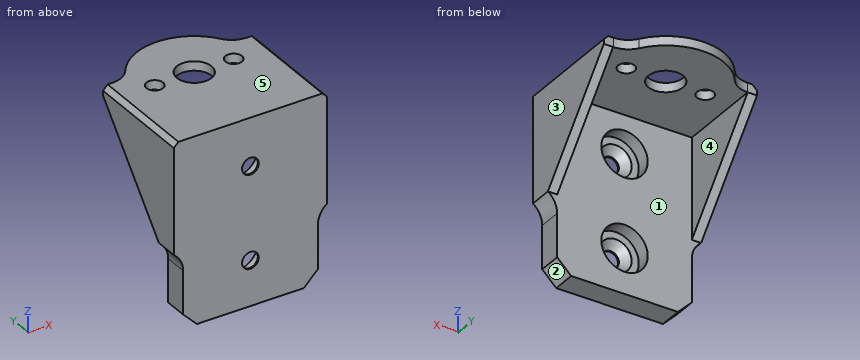
from build123d import *

# Parameters (mm, degrees)
SKETCH1_W                                    = 23
SKETCH1_H                                    = 40
SKETCH1_R                                    = 1.75
BOSS_EXTRUDE1_DEPTH                          = 5
SKETCH2_W                                    = 23
SKETCH2_H                                    = 2
BOSS_EXTRUDE2_DEPTH                          = 50
SKETCH3_R                                    = 1.8
SKETCH3_R_2                                  = 3.75
CUT_EXTRUDE1_DEPTH                           = 69.972820734
BOSS_EXTRUDE3_DEPTH                          = 3
BOSS_EXTRUDE4_START                          = -23
BOSS_EXTRUDE4_DEPTH                          = 3
BOSS_EXTRUDE5_DEPTH                          = 2
BOSS_EXTRUDE6_START                          = -29
BOSS_EXTRUDE6_DEPTH                          = 2
SKETCH6_R                                    = 5
CUT_EXTRUDE2_DEPTH                           = 3
CSK_FOR_M3_HEX_SOCKET_COUNTERSUNK_HE_2_COUNT = 2
CSK_FOR_M3_HEX_SOCKET_COUNTERSUNK_HE_2_PITCH = 20
CHAMFER1_SIZE                                = 3
CHAMFER2_SIZE                                = 1
FILLET1_R                                    = 5


with BuildPart() as part:
    # Sketch1 → Boss-Extrude1 (new body)
    with BuildSketch(Plane(origin=(0, 0, 0), x_dir=(1, 0, 0), z_dir=(0, 1, 0))):
        with Locations((0, -10.3)):
            Rectangle(SKETCH1_W, SKETCH1_H)
        with Locations(Location((0, 0, 0), (0, 0, 270))):
            Circle(SKETCH1_R, mode=Mode.SUBTRACT)
        with Locations(Location((0, -20, 0), (0, 0, 270))):
            Circle(SKETCH1_R, mode=Mode.SUBTRACT)
    extrude(amount=BOSS_EXTRUDE1_DEPTH)

    # Sketch2 → Boss-Extrude2 (add)
    with BuildSketch(Plane(origin=(0, 5, 0), x_dir=(1, 0, 0), z_dir=(0, 1, 0))):
        with Locations((0, -29.3)):
            Rectangle(SKETCH2_W, SKETCH2_H)
    extrude(amount=BOSS_EXTRUDE2_DEPTH)

    # Sketch3 → Cut-Extrude1 (cut, through all)
    with BuildSketch(Plane.XY.offset(30.3)):
        with Locations((-8.5, 18.8)):
            Circle(SKETCH3_R)
        with Locations((8.5, 18.8)):
            Circle(SKETCH3_R)
        with Locations((0, 18.8)):
            Circle(SKETCH3_R_2)
        with BuildLine():
            Line((-11.5, 23.698979486), (-11.5, 55))
            Line((-11.5, 55), (11.5, 55))
            Line((11.5, 55), (11.5, 23.698979486))
            ThreePointArc((11.5, 23.698979486), (0, 31.3), (-11.5, 23.698979486))
        make_face()
    extrude(amount=-CUT_EXTRUDE1_DEPTH, mode=Mode.SUBTRACT)

    # Sketch4 → Boss-Extrude3 (add)
    with BuildSketch(Plane.ZY.offset(11.5)):
        Polygon((30.3, 0), (30.3, 23.698979486), (28.3, 23.698979486), (28.3, 5), (-9.7, 5), (-9.7, 0), align=None)
    extrude(amount=BOSS_EXTRUDE3_DEPTH)

    # Sketch4<2> → Boss-Extrude4 (add)
    with BuildSketch(Plane.ZY.offset(11.5).offset(BOSS_EXTRUDE4_START)):
        Polygon((30.3, 0), (30.3, 23.698979486), (28.3, 23.698979486), (28.3, 5), (-9.7, 5), (-9.7, 0), align=None)
    extrude(amount=-BOSS_EXTRUDE4_DEPTH)

    # Sketch5 → Boss-Extrude5 (add)
    with BuildSketch(Plane(origin=(14.5, 0, 0), x_dir=(0, 0, -1), z_dir=(1, 0, 0))):
        Polygon((-30.3, 23.698979486), (-30.3, 0), (-6.601020514, 0), (-6.601020514, 5), (-28.3, 23.698979486), align=None)
    extrude(amount=BOSS_EXTRUDE5_DEPTH)

    # Sketch5<2> → Boss-Extrude6 (add)
    with BuildSketch(Plane(origin=(14.5, 0, 0), x_dir=(0, 0, -1), z_dir=(1, 0, 0)).offset(BOSS_EXTRUDE6_START)):
        Polygon((-30.3, 23.698979486), (-30.3, 0), (-6.601020514, 0), (-6.601020514, 5), (-28.3, 23.698979486), align=None)
    extrude(amount=-BOSS_EXTRUDE6_DEPTH)

    # Sketch6 → Cut-Extrude2 (cut)
    with BuildSketch(Plane(origin=(0, 5, 0), x_dir=(1, 0, 0), z_dir=(0, 1, 0))):
        with Locations(Location((0, 0, 0), (0, 0, 270))):
            Circle(SKETCH6_R)
        with Locations(Location((0, -20, 0), (0, 0, 270))):
            Circle(SKETCH6_R)
    extrude(amount=-CUT_EXTRUDE2_DEPTH, mode=Mode.SUBTRACT)

    # Sketch8 → CSK for M3 Hex Socket Countersunk Head Screw1 (revolve, cut)
    with BuildSketch(Plane(origin=(0, 2, 0), x_dir=(0, 0, 1), z_dir=(1, 0, 0))):
        Polygon((0, 0), (0, 2), (1.8, 2), (1.8, 1.67), (3.47, 0), align=None)
    csk_for_m3_hex_socket_countersunk_head_s = revolve(axis=Axis((0, 8.35, 0), (0, -1, 0)), mode=Mode.SUBTRACT)

    # CSK for M3 Hex Socket Countersunk He 2: CSK for M3 Hex Socket Countersunk Head Screw1 ×2
    with Locations(*[(0, 0, i * CSK_FOR_M3_HEX_SOCKET_COUNTERSUNK_HE_2_PITCH) for i in range(1, CSK_FOR_M3_HEX_SOCKET_COUNTERSUNK_HE_2_COUNT)]):
        add(csk_for_m3_hex_socket_countersunk_head_s, mode=Mode.SUBTRACT)

    # Chamfer1
    chamfer1_edges = [part.edges().sort_by_distance(p)[0] for p in [
        (-14.5, 2.5, -9.7),
        (14.5, 2.5, -9.7),
    ]]
    chamfer(chamfer1_edges, length=CHAMFER1_SIZE)

    # Chamfer2
    chamfer2_edges = [part.edges().sort_by_distance(p)[0] for p in [
        (16.5, 11.849489743, 30.3),
        (-16.5, 11.849489743, 30.3),
    ]]
    chamfer(chamfer2_edges, length=CHAMFER2_SIZE)

    # Fillet1
    # the kernel refuses this fillet: 5 mm, written as the material it adds along each edge
    with BuildSketch(Plane(origin=(11.5, 23.698979486, 30.3), x_dir=(1, 0, 0), z_dir=(0, 0, -1))) as fillet1_piece_1:
        with BuildLine():
            CenterArc((2.931223273, -5), FILLET1_R, 90, 55.552144514)
            ThreePointArc((-1.191983377, -2.171720147), (-0.54205816, -1.115462354), (0, 0))
            Line((0, 0), (2.931223273, 0))
        make_face()
    extrude(amount=2)
    with BuildSketch(Plane(origin=(-11.5, 23.698979486, 30.3), x_dir=(-1, 0, 0), z_dir=(0, 0, -1))) as fillet1_piece_2:
        with BuildLine():
            CenterArc((2.931223273, 5), FILLET1_R, 214.447855486, 55.552144514)
            ThreePointArc((-1.191983377, 2.171720147), (-0.54205816, 1.115462354), (0, 0))
            Line((0, 0), (2.931223273, 0))
        make_face()
    extrude(amount=2)
    with BuildSketch(Plane(origin=(-14.5, 0, 6.601020514), x_dir=(-1, 0, 0), z_dir=(0, 1, 0))) as fillet1_piece_3:
        with BuildLine():
            CenterArc((5, -4), FILLET1_R, 126.869897646, 53.130102354)
            Line((0, -4), (0, 0))
            Line((0, 0), (2, 0))
        make_face()
    extrude(amount=5)
    with BuildSketch(Plane(origin=(14.5, 0, 6.601020514), x_dir=(1, 0, 0), z_dir=(0, 1, 0))) as fillet1_piece_4:
        with BuildLine():
            CenterArc((5, 4), FILLET1_R, 180, 53.130102354)
            Line((0, 4), (0, 0))
            Line((0, 0), (2, 0))
        make_face()
    extrude(amount=5)


solid = part.part
Read the model definition and answer for the solid it produces. Units are mm, in the model's axes. Face numbers are marked on the shaded views. A direction names the side the tool comes from. Give positions to 0.01 mm unless a question says otherwise; leave off trailing zeros. Write each loop counter-clockwise with the first axis right and the second up, starting at its lowest first coordinate (ties: lowest second). Pieces come first, ordered by that corner, then holes. Notation, with made-up numbers: (-26, 27) -> (17, 27) arc R28 cw to (17, 58) -> close; hole circle Ø11 at (74.25, 4.25). An arc over 180 degrees is marked (long way). Answer as a JSON object with one key per item and string values. Group by question number.
1) Find section A-A (y = 18.8). Write down the section's boundary in (x, z), and give its area (3 significant figures).
2) Find section D-D (z = 13.5). Write down the section's boundary in (x, y).
3) Find section B-B (x = 8.5). Write down the section's boundary in (y, z), and give its area (3 significant figures).
4) Consider L1, parallel to Z at x = 0, y = 0.2; L2, parallel to X at y = 0.15, z = 0; L3, parallel to Z at x = -2.5, y = 2.5. Determine where each line is inside the solid, lowest interval first. Write a range as from..to.
5) A tool of negligible diameter and unlimited length cuts with its end or side. For the marked faces 1 and 2, from which of +Z, -Z, +X, -X, +Y, -Y can it reach the whole face along a straight path? Write none if from no direction.
6) The mould has two halves that part along X. Classify the marked faces 3, 4 and 5: +X half, -X half, draft (parallel to the pull), parting line (faces both ways), or undercut.
7) Find section C-C (z = 20). Write down the section's boundary in (x, y).
8) Each of these flat-tipped pins is pushed along its axis until it touches: P1, Ø2, axis at x = 15, z = 29.5, coming from the +Y side; P2, Ø5.5, axis at y = 3.5, z = -2.5, coming from the +X side; P3, Ø3, axis at x = 8.5, y = 18.8, coming from the -Z side; P4, Ø6, axis at x = 4, y = 22.5, coming from the -Z side. Where does it stop, or does it pass through?
Values follow:
{
 "1": {"outline": "(-16.5, 22.62) -> (-14.5, 22.62) -> (-14.5, 28.3) -> (-10.3, 28.3) -> (-10.3, 30.3) -> (-15.5, 30.3) -> (-16.5, 29.3) -> close; (-6.7, 28.3) -> (-3.75, 28.3) -> (-3.75, 30.3) -> (-6.7, 30.3) -> close; (3.75, 28.3) -> (6.7, 28.3) -> (6.7, 30.3) -> (3.75, 30.3) -> close; (10.3, 28.3) -> (14.5, 28.3) -> (14.5, 22.62) -> (16.5, 22.62) -> (16.5, 29.3) -> (15.5, 30.3) -> (10.3, 30.3) -> close", "area": "58.3 mm2"},
 "2": {"outline": "(-16.5, 0) -> (16.5, 0) -> (16.5, 10.95) -> (14.5, 10.95) -> (14.5, 5) -> (-14.5, 5) -> (-14.5, 10.95) -> (-16.5, 10.95) -> close"},
 "3": {"outline": "(0, -9.7) -> (5, -9.7) -> (5, 28.3) -> (17, 28.3) -> (17, 30.3) -> (0, 30.3) -> close; (20.6, 28.3) -> (27.97, 28.3) -> (27.97, 30.3) -> (20.6, 30.3) -> close", "area": "239 mm2"},
 "4": {"L1": "z = -9.7..-1.8, 1.8..18.2, 21.8..30.3", "L2": "x = -14.5..-1.8, 1.8..14.5", "L3": "z = -9.7..-4.33, 4.33..15.67, 24.33..30.3"},
 "5": {"face 1": "-Z, +Y", "face 2": "-Z, +X, +Y, -Y"},
 "6": {"face 3": "+X half", "face 4": "undercut", "face 5": "draft"},
 "7": {"outline": "(-16.5, 0) -> (-1.8, 0) -> (-1.8, 0.33) -> (-3.47, 2) -> (-5, 2) -> (-5, 5) -> (-14.5, 5) -> (-14.5, 16.55) -> (-16.5, 16.55) -> close; (1.8, 0) -> (16.5, 0) -> (16.5, 16.55) -> (14.5, 16.55) -> (14.5, 5) -> (5, 5) -> (5, 2) -> (3.47, 2) -> (1.8, 0.33) -> close"},
 "8": {"P1": "stops at y = 23.72", "P2": "stops at x = 14.5", "P3": "passes through", "P4": "stops at z = 28.3"}
}
